```python
from build123d import *

# Parameters (mm, degrees)
EXTRUDE_4_DEPTH     = 1
EXTRUDE_5_DEPTH     = 2.5
CUT_EXTRUDE_2_DEPTH = 30.837057496
SKETCH_6_R          = 3
CUT_EXTRUDE_3_DEPTH = 30.837057496
SKETCH_7_W          = 38
SKETCH_7_H          = 2.5
CUT_EXTRUDE_4_DEPTH = 47.650294747
EXTRUDE_6_DEPTH     = 2.5


with BuildPart() as part:
    # 草图1 → 凸台-拉伸4 (new body)
    with BuildSketch(Plane(origin=(0, 0, 0), x_dir=(1, 0, 0), z_dir=(0, 1, 0))):
        with BuildLine():
            ThreePointArc((20, 0), (0, 20), (-20, 0))
            Line((-20, 0), (20, 0))
        make_face()
        with BuildLine():
            Line((20, 0), (-20, 0))
            ThreePointArc((-20, 0), (0, -20), (20, 0))
        make_face()
        with BuildLine():
            ThreePointArc((20, 0), (0, -20), (-20, 0))
            Line((-20, 0), (-20, -22))
            Line((-20, -22), (20, -22))
            Line((20, -22), (20, 0))
        make_face()
    extrude(amount=EXTRUDE_4_DEPTH)

    # 草图4 → 凸台-拉伸5 (add)
    with BuildSketch(Plane(origin=(0, 1, 0), x_dir=(1, 0, 0), z_dir=(0, 1, 0))):
        with BuildLine():
            ThreePointArc((20, 0), (0, -20), (-20, 0))
            Line((-20, 0), (-20, -22))
            Line((-20, -22), (20, -22))
            Line((20, -22), (20, 0))
        make_face()
    extrude(amount=EXTRUDE_5_DEPTH)

    # 草图5 → 切除-拉伸2 (cut, through all)
    with BuildSketch(Plane(origin=(0, 1, 0), x_dir=(1, 0, 0), z_dir=(0, 1, 0))):
        with BuildLine():
            ThreePointArc((-7.251630242, -3.378440296), (-6.92820323, 4), (-0.7, 7.969316156))
            Line((-0.7, 7.969316156), (-0.7, 18.987100885))
            ThreePointArc((-0.7, 18.987100885), (-16.454482672, 9.5), (-16.79331171, -8.88733266))
            Line((-16.79331171, -8.88733266), (-7.251630242, -3.378440296))
        make_face()
        with BuildLine():
            ThreePointArc((8, 0), (7.810667127, -1.730167342), (7.251630242, -3.378440296))
            Line((7.251630242, -3.378440296), (16.79331171, -8.88733266))
            ThreePointArc((16.79331171, -8.88733266), (18.440077582, -4.578595718), (19, 0))
            ThreePointArc((19, 0), (13.680277775, 13.185218997), (0.7, 18.987100885))
            Line((0.7, 18.987100885), (0.7, 7.969316156))
            ThreePointArc((0.7, 7.969316156), (5.899152482, 5.403702434), (8, 0))
        make_face()
        with BuildLine():
            Line((16.09331171, -10.099768225), (6.551630242, -4.590875861))
            ThreePointArc((6.551630242, -4.590875861), (0, -8), (-6.551630242, -4.590875861))
            Line((-6.551630242, -4.590875861), (-16.09331171, -10.099768225))
            ThreePointArc((-16.09331171, -10.099768225), (0, -19), (16.09331171, -10.099768225))
        make_face()
    extrude(amount=-CUT_EXTRUDE_2_DEPTH, mode=Mode.SUBTRACT)

    # 草图6 → 切除-拉伸3 (cut, through all)
    with BuildSketch(Plane(origin=(0, 1, 0), x_dir=(1, 0, 0), z_dir=(0, 1, 0))):
        with Locations(Location((0, 0, 0), (0, 0, 270))):
            Circle(SKETCH_6_R)
    extrude(amount=-CUT_EXTRUDE_3_DEPTH, mode=Mode.SUBTRACT)

    # 草图7 → 切除-拉伸4 (cut, through all)
    with BuildSketch(Plane.XY.offset(22)):
        with Locations((0, 2.25)):
            Rectangle(SKETCH_7_W, SKETCH_7_H)
    extrude(amount=-CUT_EXTRUDE_4_DEPTH, mode=Mode.SUBTRACT)

    # 草图8 → 凸台-拉伸6 (add)
    with BuildSketch(Plane(origin=(0, 1, 0), x_dir=(1, 0, 0), z_dir=(0, 1, 0))):
        Polygon((19, -14.122498999), (13.960934911, -22), (19, -22), align=None)
        Polygon((-19, -14.122498999), (-14.007707412, -22), (-19, -22), align=None)
    extrude(amount=EXTRUDE_6_DEPTH)


solid = part.part
```
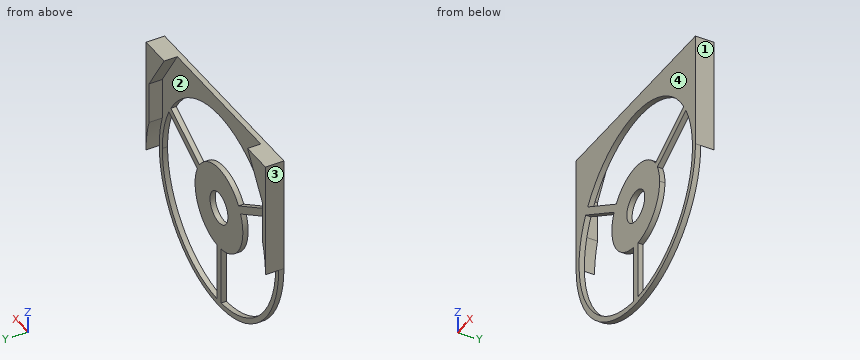
Check sheet for the modelled part. Datum: model origin and axes. Units: mm. Face numbers are marked on the shaded views. Coordinates: 2 decimals unless noted, no trailing zeros. Order: outer loops, then holes, each group sorted by start corner. A loop starts at its lowest first (then second) coordinate and runs counter-clockwise, first axis right, second up. Notation, with made-up numbers: (26.25, 53) -> (58.25, 53) arc R25 ccw to (58.25, 79) -> close; hole circle Ø7 at (59.5, -2.5). An arc over 180 degrees is marked (long way). Write item = value, one per line. Start each with the question number.
1) Cross-section at D-D (z = 16.5). Enter the section's corners in (x, y).
2) Go/stop test with flat-tipped pins: P1, Ø0.8, axis at y = 0.5, z = -13, coming from the -X side; P2, Ø20, axis at x = -6.5, z = 0.5, coming from the +Y side; P3, Ø1.1, axis at y = 0.5, z = -11.5, coming from the +X side. Record where each tip stops, or that it passes through.
3) Cross-section at A-A (y = 2). Enter the section's corners in (x, z) (1 decimal), then the cut area to 3 significant figures.
4) Cross-section at C-C (x = 0). Enter the section's corners in (y, z).
5) Cross-section at B-B (z = -0.5). Enter the section's corners in (x, y), then the cut area to 3 significant figures.
6) Mould release check, pull along X, two halves, no side actions. Record for the marked faces 1, 2, 3 and 4: +X half, -X half, draft (parallel to the pull), parting line (faces both ways), or undercut.
7) Material ranges on L1, parallel to X at y = 0.75, z = 0; L2, parallel to X at y = 0.4, z = 2.5; L3, parallel to X at y = 0.2, z = -8, recorded low to high.
Ans:
q1.outline = (-20, 0) -> (-9.42, 0) -> (-9.42, 1) -> (-17.49, 1) -> (-17.49, 3.5) -> (-20, 3.5) -> close; (9.42, 0) -> (20, 0) -> (20, 3.5) -> (17.48, 3.5) -> (17.48, 1) -> (9.42, 1) -> close
q2.P1 = -15.53
q2.P2 = 1
q2.P3 = 16.74
q3.outline = (-20, 0) arc R20 cw to (-19, 6.2) -> (-19, 14.1) -> (-14, 22) -> (-20, 22) -> close; (14, 22) -> (19, 14.1) -> (19, 6.2) arc R20 cw to (20, 0) -> (20, 22) -> close
q3.area = 75.1 mm²
q4.outline = (0, -20) -> (1, -20) -> (1, -3) -> (0, -3) -> close; (0, 3) -> (1, 3) -> (1, 8) -> (0, 8) -> close; (0, 19) -> (1, 19) -> (1, 22) -> (0, 22) -> close
q5.outline = (-19.99, 0) -> (-18.99, 0) -> (-18.99, 1) -> (-19.99, 1) -> close; (-7.98, 0) -> (-2.96, 0) -> (-2.96, 1) -> (-7.98, 1) -> close; (2.96, 0) -> (7.98, 0) -> (7.98, 1) -> (2.96, 1) -> close; (18.99, 0) -> (19.99, 0) -> (19.99, 1) -> (18.99, 1) -> close
q5.area = 12.1 mm²
q6.face_1 = +X half
q6.face_2 = undercut
q6.face_3 = -X half
q6.face_4 = draft
q7.L1 = -20 to -19, -8 to -3, 3 to 8, 19 to 20
q7.L2 = -20 to -18.83, -7.6 to -1.66, 1.66 to 7.6, 18.83 to 20
q7.L3 = -18.33 to -17.23, -0.7 to 0.7, 17.23 to 18.33
